```python
from build123d import *

# Parameters (mm, degrees)
BOSS_EXTRUDE1_DEPTH                                 = 4
CSK_FOR_M3_COUNTERSUNK_FLAT_HEAD_SCREW1_D           = 3.4
CSK_FOR_M3_COUNTERSUNK_FLAT_HEAD_SCREW1_CSINK_D     = 6.3
CSK_FOR_M3_COUNTERSUNK_FLAT_HEAD_SCREW1_CSINK_ANGLE = 90
CSK_FOR_M3_COUNTERSUNK_FLAT_HEAD_SCREW2_D           = 3.4
CSK_FOR_M3_COUNTERSUNK_FLAT_HEAD_SCREW2_CSINK_D     = 6.3
CSK_FOR_M3_COUNTERSUNK_FLAT_HEAD_SCREW2_CSINK_ANGLE = 90
SKETCH7_W                                           = 1.222113554
SKETCH7_H                                           = 3.336226563
CUT_EXTRUDE1_DEPTH                                  = 4


with BuildPart() as part:
    # Sketch1 → Boss-Extrude1 (new body)
    with BuildSketch(Plane(origin=(0, 0, 0), x_dir=(1, 0, 0), z_dir=(0, 1, 0))):
        with BuildLine():
            Line((-15, -20), (15, -20))
            ThreePointArc((15, -20), (18.535533906, -18.535533906), (20, -15))
            Line((20, -15), (20, 15))
            ThreePointArc((20, 15), (18.535533906, 18.535533906), (15, 20))
            Line((15, 20), (-15, 20))
            ThreePointArc((-15, 20), (-18.535533906, 18.535533906), (-20, 15))
            Line((-20, 15), (-20, -15))
            ThreePointArc((-20, -15), (-18.535533906, -18.535533906), (-15, -20))
        make_face()
    extrude(amount=BOSS_EXTRUDE1_DEPTH)

    # CSK for M3 Countersunk Flat Head Screw1 (through all)
    with Locations(Plane(origin=(-14, 4, -14), x_dir=(0, 0, 1), z_dir=(0, 1, 0))):
        with Locations((0, 0), (0, 28), (28, 28), (28, 0)):
            CounterSinkHole(CSK_FOR_M3_COUNTERSUNK_FLAT_HEAD_SCREW1_D / 2, CSK_FOR_M3_COUNTERSUNK_FLAT_HEAD_SCREW1_CSINK_D / 2, counter_sink_angle=CSK_FOR_M3_COUNTERSUNK_FLAT_HEAD_SCREW1_CSINK_ANGLE)

    # CSK for M3 Countersunk Flat Head Screw2 (through all)
    with Locations(Plane(origin=(0, 0, 0), x_dir=(-1, 0, 0), z_dir=(0, -1, 0))):
        with Locations((3.5, -0.1976847), (3.5, -7.1976847)):
            CounterSinkHole(CSK_FOR_M3_COUNTERSUNK_FLAT_HEAD_SCREW2_D / 2, CSK_FOR_M3_COUNTERSUNK_FLAT_HEAD_SCREW2_CSINK_D / 2, counter_sink_angle=CSK_FOR_M3_COUNTERSUNK_FLAT_HEAD_SCREW2_CSINK_ANGLE)

    # Sketch7 → Cut-Extrude1 (cut)
    with BuildSketch(Plane(origin=(0, 4, 0), x_dir=(1, 0, 0), z_dir=(0, 1, 0))):
        with Locations((-11.652287397, 3.708478162)):
            Rectangle(SKETCH7_W, SKETCH7_H)
        with BuildLine():
            add(Edge.make_bspline(
                [(-15.043692162, -2.806314504), (-14.880436161, -2.741055239), (-14.5584639, -2.612351406), (-14.077627456, -2.435113354), (-13.607003536, -2.275557203), (-13.296000815, -2.177928582), (-13.143053989, -2.129916179)],
                knots=[0, 0, 0, 0, 0.000527431, 0.001040195, 0.001537166, 0.002018074, 0.002018074, 0.002018074, 0.002018074], degree=3))
            Line((-13.143053989, -2.129916179), (-13.142217189, -2.10714082))
            add(Edge.make_bspline(
                [(-13.142217189, -2.10714082), (-13.300142366, -2.053259121), (-13.613682824, -1.946283823), (-14.081290903, -1.775427697), (-14.553659216, -1.59628161), (-14.870442844, -1.470693808), (-15.032410797, -1.406482159)],
                knots=[0, 0, 0, 0, 0.000500579, 0.000993836, 0.001493443, 0.002016132, 0.002016132, 0.002016132, 0.002016132], degree=3))
            Line((-15.032410797, -1.406482159), (-17.320356965, -0.487540494))
            Line((-17.320356965, -0.487540494), (-17.320356965, 1.515068939))
            Line((-17.320356965, 1.515068939), (-11.797862272, -1.130802918))
            Line((-11.797862272, -1.130802918), (-8.007023631, -1.130802918))
            Line((-8.007023631, -1.130802918), (-8.007023631, -2.914806972))
            Line((-8.007023631, -2.914806972), (-11.858418799, -2.914806972))
            Line((-11.858418799, -2.914806972), (-17.320356965, -5.682049098))
            Line((-17.320356965, -5.682049098), (-17.320356965, -3.703713718))
            Line((-17.320356965, -3.703713718), (-15.043692162, -2.806314504))
        make_face()
    extrude(amount=-CUT_EXTRUDE1_DEPTH, mode=Mode.SUBTRACT)


solid = part.part
```
Design review of the part built by this model. Coordinates are the model's own, in mm. A direction names the side the tool comes from. Give positions to 0.01 mm unless a question says otherwise; leave off trailing zeros. Order: outer loops, then holes, each group sorted by start corner. A loop starts at its lowest first (then second) coordinate and runs counter-clockwise, first axis right, second up. Notation, with made-up numbers: (-25, -17.5) -> (33, -17.5) arc R37 ccw to (33, 19.5) -> close; hole circle Ø6 at (-15, 86). An arc over 180 degrees is marked (long way). Write item = value, one per line. Start each with the question number.
(1) We need section A-A on x = -3.5. Write out the cut boundary in (y, z).
(2) Mouldability with a two-part tool opening along X and no side actions: class faces 3 (the face through (0, 0, 0)), 4 (the face through (18, 2, 19)), 5 (the face through (14.51, 1.26, 12.38)) as +X half, -X half, draft (parallel to the pull), parting line (faces both ways), or undercut.
(3) We need section B-B on z = -14. Write out the cut boundary in (x, y).
(4) For pin 1 (3 mm diameter, centred on x = 14, z = -14.5, fed in from +Y); pin 2 (2.5 mm diameter, centred on x = 14, z = 14, fed in from +Y); pin 3 (8 mm diameter, centred on x = -11.5, z = -7, fed in from -Y), all flat-tipped, find the tip position at first contact; note any pin that passes through.
(5) For faces 1 (the face through (0, 2, -20)), 2 (the face through (-8.007, 2, 2)), list the 3-axis set-ups (+Z, -Z, +X, -X, +Y, -Y) from which the entire face can be reached by the end or side of a thin tool; tool diameter is ignored.
(6) We need section C-C on y = 2.05. State how many separate pieces and enclosed holes the cut face has, plus the area to 3 significant figures.
(7) To check wall thickness, follow line 1 along Z through (x, y) = (14, 0.65); line 2 along Z through (x, y) = (-3.5, 2.45). State the ranges of each line that lie inside material, in increasing order.
Numbers:
q1.outline = (0, -20) -> (4, -20) -> (4, -1.5) -> (1.45, -1.5) -> (0, -2.95) -> close; (0, 3.35) -> (1.45, 1.9) -> (4, 1.9) -> (4, 5.5) -> (1.45, 5.5) -> (0, 4.05) -> close; (0, 10.35) -> (1.45, 8.9) -> (4, 8.9) -> (4, 20) -> (0, 20) -> close
q2.face_3 = draft
q2.face_4 = +X half
q2.face_5 = undercut
q3.outline = (-20, 0) -> (-15.7, 0) -> (-15.7, 2.55) -> (-17.15, 4) -> (-20, 4) -> close; (-12.3, 0) -> (12.3, 0) -> (12.3, 2.55) -> (10.85, 4) -> (-10.85, 4) -> (-12.3, 2.55) -> close; (15.7, 0) -> (20, 0) -> (20, 4) -> (17.15, 4) -> (15.7, 2.55) -> close
q4.pin_1 = 2.85
q4.pin_2 = through
q4.pin_3 = 0
q5.face_1 = -Z, +X, -X, +Y, -Y
q5.face_2 = +Y, -Y
q6.separate_pieces = 1
q6.enclosed_holes = 8
q6.area = 1,500 mm^2
q7.line_1 = -20 to -15.7, -12.3 to 12.3, 15.7 to 20
q7.line_2 = -20 to -1.5, 1.9 to 5.5, 8.9 to 20
